Part model, mm, in its own coordinate system. Face numbers are marked on the shaded views. Round coordinates to 2 decimals unless told otherwise and drop trailing zeros. Loops run counter-clockwise (first coordinate to the right, second up) from the corner with the lowest first, then second, coordinate; pieces in that order, holes last. Notation, with made-up numbers: M 69,35.25 L 106,35.25 A30 cw 106,74.25 Z; hole C 38.5,47 d8. An arc over 180 degrees is marked long. Put each result on its own line as item: value. Start each with the question number.
```python
from build123d import *

# Parameters (mm, degrees)
SKETCH2_W           = 101.6
SKETCH2_H           = 280
BOSS_EXTRUDE1_DEPTH = 25.4
SKETCH3_R           = 6.75
SKETCH3_R_2         = 41.5
CUT_EXTRUDE1_DEPTH  = 25.4
SKETCH4_R           = 5.25
CUT_EXTRUDE2_DEPTH  = 25.4


with BuildPart() as part:
    # Sketch2 → Boss-Extrude1 (new body)
    with BuildSketch(Plane(origin=(0, 0, 0), x_dir=(1, 0, 0), z_dir=(0, 1, 0))):
        with Locations((50.8, 140)):
            Rectangle(SKETCH2_W, SKETCH2_H)
    extrude(amount=BOSS_EXTRUDE1_DEPTH)

    # Sketch3 → Cut-Extrude1 (cut)
    with BuildSketch(Plane(origin=(0, 25.4, 0), x_dir=(1, 0, 0), z_dir=(0, 1, 0))):
        with Locations((71, 245)):
            Circle(SKETCH3_R)
        with Locations((31, 245)):
            Circle(SKETCH3_R)
        with Locations((71, 145)):
            Circle(SKETCH3_R)
        with Locations((31, 145)):
            Circle(SKETCH3_R)
        with Locations((51, 195)):
            Circle(SKETCH3_R_2)
    extrude(amount=-CUT_EXTRUDE1_DEPTH, mode=Mode.SUBTRACT)

    # Sketch4 → Cut-Extrude2 (cut)
    with BuildSketch(Plane(origin=(0, 25.4, 0), x_dir=(1, 0, 0), z_dir=(0, 1, 0))):
        with Locations((71, 105)):
            Circle(SKETCH4_R)
        with Locations((31, 105)):
            Circle(SKETCH4_R)
        with Locations((31, 25)):
            Circle(SKETCH4_R)
        with Locations((71, 25)):
            Circle(SKETCH4_R)
    extrude(amount=-CUT_EXTRUDE2_DEPTH, mode=Mode.SUBTRACT)


solid = part.part
```
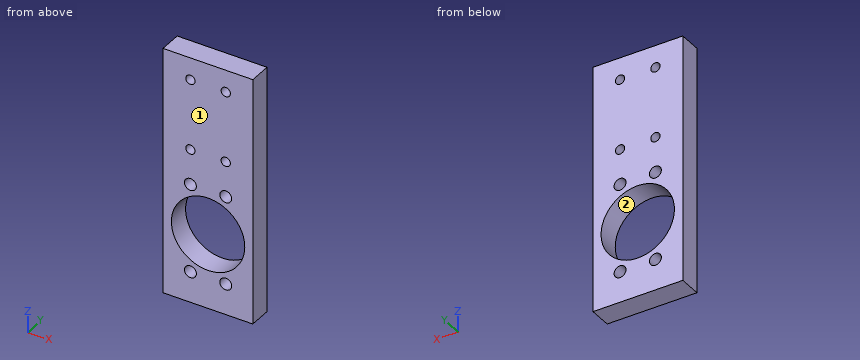
1. Cut at B-B, the plane x = 51. Give the cut face in (y, z), and give its area (3 significant figures).
2. Cut at C-C, the plane z = -195. Give the cut face in (x, y), and give its area (3 significant figures).
3. Drop a flat-ended pin along its axis: pin 1 (12 mm diameter, centred on x = 71, z = -105, fed in from +Y). Give the stop position or say it passes through.
4. Mould opens along X. For the marked faces 1 and 2 say: released by +X, released by -X, zero draft, split by the parting line, or undercut.
5. Wall check: L1, parallel to X at y = 19.5, z = -145; L2, parallel to X at y = 14.75, z = -25; L3, parallel to Z at x = 71, y = 10. Give the ranges that are in metal, low to high.
6. Cut at A-A, the plane z = -245. Give the cut face in (x, y).
7. Cut at D-D, the plane y = 17. Give the number of separate pieces and of enclosed holes in the cut face, and give its area (3 significant figures).
Results list:
1. outline: M 0,-280 L 25.4,-280 L 25.4,-236.5 L 0,-236.5 Z; M 0,-153.5 L 25.4,-153.5 L 25.4,0 L 0,0 Z
1. area: 5,000 mm^2
2. outline: M 0,0 L 9.5,0 L 9.5,25.4 L 0,25.4 Z; M 92.5,0 L 101.6,0 L 101.6,25.4 L 92.5,25.4 Z
2. area: 472 mm^2
3. pin 1: stops at y = 25.4
4. face 1: zero draft
4. face 2: undercut
5. L1: x = 0 to 24.25, 37.75 to 64.25, 77.75 to 101.6
5. L2: x = 0 to 25.75, 36.25 to 65.75, 76.25 to 101.6
5. L3: z = -280 to -251.75, -238.25 to -231.36, -158.64 to -151.75, -138.25 to -110.25, -99.75 to -30.25, -19.75 to 0
6. outline: M 0,0 L 24.25,0 L 24.25,25.4 L 0,25.4 Z; M 37.75,0 L 64.25,0 L 64.25,25.4 L 37.75,25.4 Z; M 77.75,0 L 101.6,0 L 101.6,25.4 L 77.75,25.4 Z
7. separate pieces: 1
7. enclosed holes: 9
7. area: 22,100 mm^2
